```python
from build123d import *

# Parameters (mm, degrees)
F2_SIZE  = 2
F3_R     = 23.495
F3_R_2   = 22.86
F4_DEPTH = 2


with BuildPart() as f1:
    # F0 (on Top) → F1 (revolve)
    with BuildSketch(Plane.XY):
        Polygon((0, 3), (0, 0), (25.4, 0), (25.4, 3), (19.936919, 3), (19.936919, 2.25), (18.997, 2.25), (18.997, 2.5), (18.75, 2.5), (18.75, 2.75), (18.5, 2.75), (18.5, 3), (18.246, 3), (18.246, 2.25), (17.989, 2.25), (17.989, 2.5), (17.728, 2.5), (17.728, 2.75), (17.463, 2.75), (17.463, 3), (17.194, 3), (17.194, 2.25), (16.922, 2.25), (16.922, 2.5), (16.645, 2.5), (16.645, 2.75), (16.363, 2.75), (16.363, 3), (16.077, 3), (16.077, 2.25), (15.785, 2.25), (15.785, 2.5), (15.488, 2.5), (15.488, 2.75), (15.186, 2.75), (15.186, 3), (14.877, 3), (14.877, 2.25), (14.562, 2.25), (14.562, 2.5), (14.241, 2.5), (14.241, 2.75), (13.912, 2.75), (13.912, 3), (13.575, 3), (13.575, 2.25), (13.23, 2.25), (13.23, 2.5), (12.875, 2.5), (12.875, 2.75), (12.510997, 2.75), (12.510997, 3), (12.136, 3), (12.136, 2.25), (11.749, 2.25), (11.749, 2.5), (11.35, 2.5), (11.35, 2.75), (10.936, 2.75), (10.936, 3), (10.505, 3), (10.505, 2.25), (10.057, 2.25), (10.057, 2.5), (9.588, 2.5), (9.588, 2.75), (9.095, 2.75), (9.095, 3), (8.584906, 3), (8.573998, 2.25), (8.019, 2.25), (8.019, 2.5), (7.423, 2.5), (7.423, 2.75), (6.776, 2.75), (6.776, 3), (6.06, 3), (6.06, 2.25), (5.247, 2.25), (5.247, 2.5), (4.284, 2.5), (4.284, 2.75), (3.029, 2.75), (3.029, 3), align=None)
    revolve(axis=Axis((0, 1.5, 0), (0, 1, 0)))

    # F2
    f2_edges = [f1.edges().sort_by_distance(p)[0] for p in [
        (-25.4, 0, 0),
    ]]
    chamfer(f2_edges, length=F2_SIZE)

    # F3 (on Front) → F4 (join)
    with BuildSketch(Plane.XZ):
        Circle(F3_R)
        Circle(F3_R_2, mode=Mode.SUBTRACT)
    extrude(amount=F4_DEPTH)


solid = f1.part
```
Here's how the part is built. I have some questions about the finished solid (model axes, mm). A direction names the side the tool comes from. Coordinates: 2 decimals unless noted, no trailing zeros. Order: outer loops, then holes, each group sorted by start corner. A loop starts at its lowest first (then second) coordinate and runs counter-clockwise, first axis right, second up. Notation, with made-up numbers: (43, -16.5) - (67, -16.5) arc R28 ccw to (67, 8.5) - close; hole circle Ø9 at (16.5, 76.25). An arc over 180 degrees is marked (long way). One line per question, with ' | ' between items.
(1) If I drill on L1, parallel to Z at x = -15.5, y = -1.35; L2, parallel to Y at x = -8, z = -13.5; L3, parallel to Z at x = 8.5, y = -0.25, over which ranges is the centre line in solid material (lowest first)?
Report:
L1: z = -17.66 to -16.8, 16.8 to 17.66 | L2: y = 0 to 2.5 | L3: z = -21.9 to -21.22, 21.22 to 21.9
(2) If we mould it in two halves opening along X, with no side actions, what happens to faces 3 (the flat face through (-4, 3, -10)), 4 (the flat face through (12.9, 2.5, 6.4))? For each: pulls with the +X half, pulls with the -X half, needs draft (parallel to the pull), parting line crosses it, or undercut.
Report:
face 3: needs draft | face 4: undercut
(3) For faces 1 (the cylindrical face through (15.335, 2.62, -4.829)), 2 (the flat face through (-2, 3, 6)), which set-ups out of +Z, -Z, +X, -X, +Y, -Y let a thin tool reach every point of the face, with its end or its side?
Report:
face 1: +Y | face 2: +Z, -Z, +X, -X, +Y
(4) Suppose I cut it at A-A on y = -0.6. List the corners of the cut face in (x, z) for me (3 decimals), and give its area (3 significant figures).
Report:
outline: circle Ø46.99 at (0, 0); hole circle Ø45.72 at (0, 0) | area: 92.5 mm2
(5) Will these pins go through, and if not, where does the flat tip stop? pin 1 (8 mm diameter, centred on x = -18, z = 2, fed in from -Y); pin 2 (18 mm diameter, centred on x = -2.5, z = -3.5, fed in from +Y); pin 3 (3 mm diameter, centred on y = -0.5, z = 10.5, fed in from +X); pin 4 (1 mm diameter, centred on y = -0.5, z = 6, fed in from +X).
Report:
pin 1: stops at y = 0 | pin 2: stops at y = 3 | pin 3: stops at x = 22.16 | pin 4: stops at x = 22.84
